For this review, use the dimensioned drawing (mm, ordinates from the lowest corner) and the shaded views. Coordinates: 2 decimals unless noted, no trailing zeros. Write each loop counter-clockwise with the first axis right and the second up, starting at its lowest first coordinate (ties: lowest second). Pieces come first, ordered by that corner, then holes. Notation, with made-up numbers: (-35, 18) - (0, 18) arc R18 cw to (0, 38) - close; hole circle Ø9 at (57.25, 0.25). An arc over 180 degrees is marked (long way). Put each result on its own line as item: value.
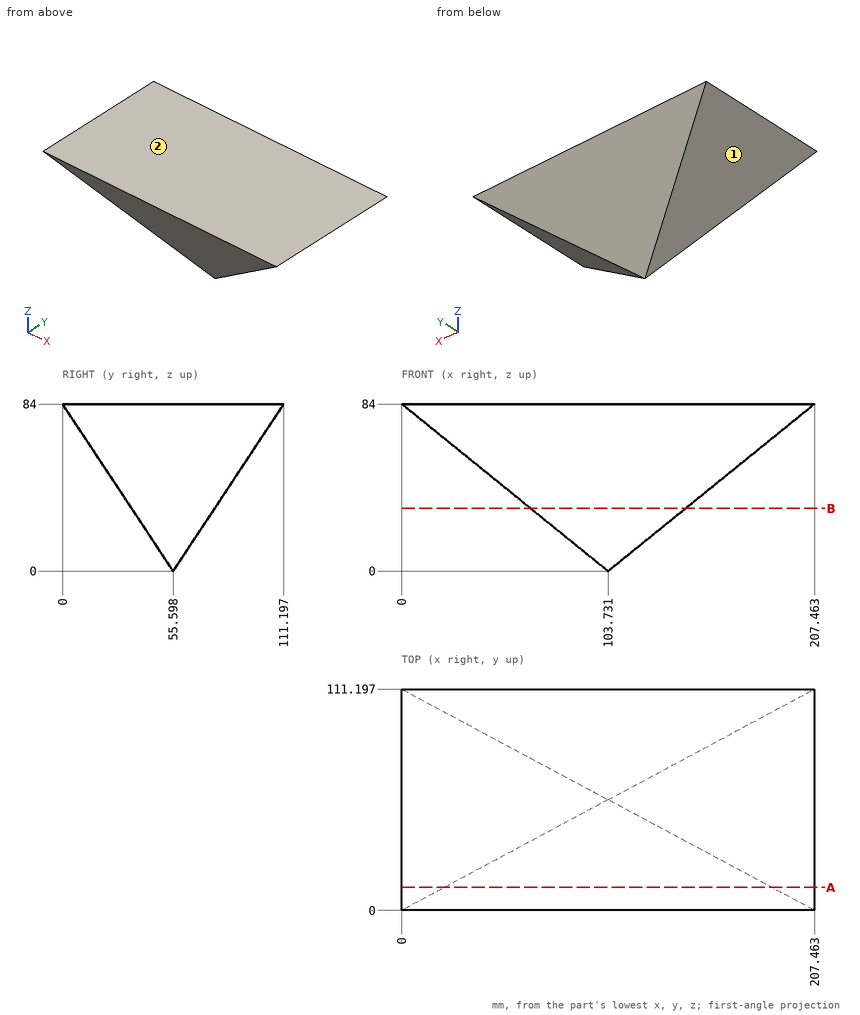
1. Consider section B-B on z = 31.5. State the section outline as (x, y) points.
Determined:
outline: (64.83, 34.75) - (142.63, 34.75) - (142.63, 76.45) - (64.83, 76.45) - close
2. For pin 1 Ø1 at (y, z) = (47.5, 29.5) entering from +X; pin 2 Ø8 at (y, z) = (46, 22.5) entering from -X (1 decimal); pin 3 Ø10 at (y, z) = (25.5, 38.5) entering from +X (1 decimal), all flat-tipped, find the tip position at first contact; note any pin that passes through.
Determined:
pin 1: stops at x = 140.78
pin 2: stops at x = 71
pin 3: stops at x = 157.2
3. The part is to be moulded in two halves that separate along X. For the marked faces 1 and 2, say which applies: +X half, -X half, draft (parallel to the pull), parting line (faces both ways), or undercut.
Determined:
face 1: -X half
face 2: draft
4. Consider section A-A on y = 11.5. State the section outline as (x, z) points (1 decimal).
Determined:
outline: (0, 84) - (21.5, 66.6) - (186, 66.6) - (207.5, 84) - close
5. To check wall thickness, follow probe 1 along Z at (x, y) = (94.5, 94); probe 2 along X at (y, z) = (65.5, 25) (1 decimal); probe 3 along Z at (x, y) = (180.5, 15.5) (1 decimal). State the ranges of each line that lie inside material, in increasing order.
Determined:
probe 1: z = 58.02 to 84
probe 2: x = 72.9 to 134.6
probe 3: z = 62.2 to 84
